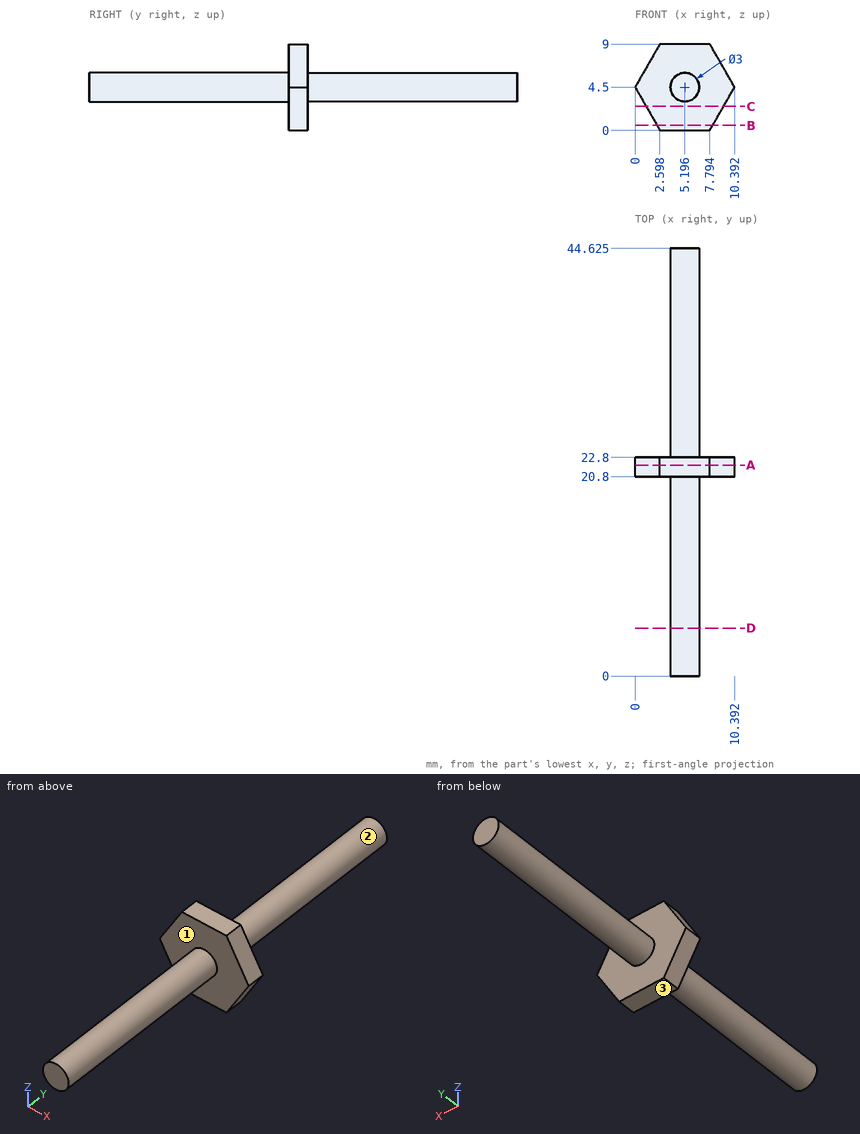
Here's the drawing with two shaded views (mm, measured from the low corner). I have some questions. A direction names the side the tool comes from. Give positions to 0.01 mm unless a question says otherwise; leave off trailing zeros. Write each loop counter-clockwise with the first axis right and the second up, starting at its lowest first coordinate (ties: lowest second). Pieces come first, ordered by that corner, then holes. Notation, with made-up numbers: (-29, -36) -> (7, -36) arc R16 ccw to (7, -9) -> close; hole circle Ø2 at (-32.75, 75.5). An arc over 180 degrees is marked (long way). Answer as a JSON object with one key per item and string values. Group by question number.
Item 1: Please list where these lines run through material, in increasing order: line 1 (Y direction, x = 2.5, z = 1.25); line 2 (Z direction, x = 4, y = 23) (1 decimal); line 3 (X direction, y = 21.5, z = 7.25) (1 decimal). Write a range as [from, to].
Item 2: Suppose I cut it at A-A (y = 22). Please give me the cut outline in (x, z).
Item 3: For the marked faces 1, 2 and 3, which set-ups out of +Z, -Z, +X, -X, +Y, -Y let a thin tool reach every point of the face, with its end or its side?
Item 4: Suppose I cut it at B-B (z = 0.5). Please give me the cut outline in (x, y).
Item 5: Suppose I cut it at C-C (z = 2.5). Please give me the cut outline in (x, y) (1 decimal), plus the area to 3 significant figures.
Item 6: Suppose I cut it at D-D (y = 5). Please give me the cut outline in (x, z).
Item 7: I'm going to push a flat-ended pin straight in: P1, Ø1, axis at x = 4, y = 14.5, coming from the +Z side. Where does the tip first touch, or does it pass through?
Findings:
{
 "1": {"line 1": "y = [20.8, 22.8]", "line 2": "z = [3.6, 5.4]", "line 3": "x = [1.6, 8.8]"},
 "2": {"outline": "(0, 4.5) -> (2.6, 0) -> (7.79, 0) -> (10.39, 4.5) -> (7.79, 9) -> (2.6, 9) -> close"},
 "3": {"face 1": "-Y", "face 2": "+Y", "face 3": "-Z, +X, -X, +Y, -Y"},
 "4": {"outline": "(2.31, 20.8) -> (8.08, 20.8) -> (8.08, 22.8) -> (2.31, 22.8) -> close"},
 "5": {"outline": "(1.2, 20.8) -> (9.2, 20.8) -> (9.2, 22.8) -> (1.2, 22.8) -> close", "area": "16.2 mm²"},
 "6": {"outline": "circle Ø3 at (5.2, 4.5)"},
 "7": {"P1": "stops at z = 5.83"}
}
